Source: CAD feature listing. Evaluate the final solid. Frame: model axes, mm. Face numbers are marked on the shaded views. A direction names the side the tool comes from. Round coordinates to 2 decimals unless told otherwise and drop trailing zeros. Write each loop counter-clockwise with the first axis right and the second up, starting at its lowest first coordinate (ties: lowest second). Pieces come first, ordered by that corner, then holes.
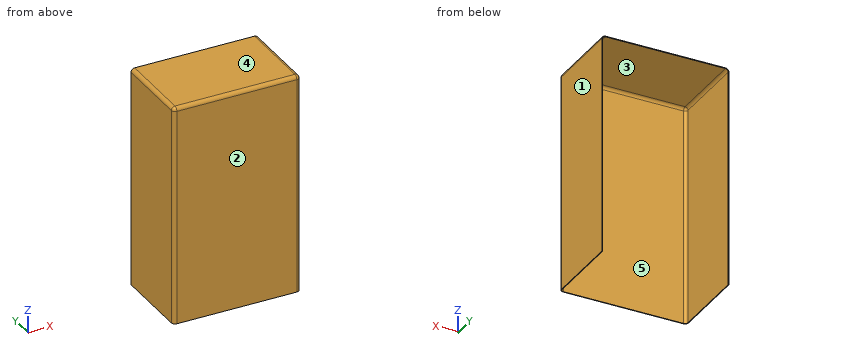
```python
from build123d import *

# Parameters (mm, degrees)
SKETCH_1_W      = 350
SKETCH_1_H      = 220
EXTRUDE_1_DEPTH = 607
FILLET_1_R      = 10
SHELL_1_T       = -2


with BuildPart() as part:
    # 草图1 → 凸台-拉伸1 (new body)
    with BuildSketch(Plane.XY):
        Rectangle(SKETCH_1_W, SKETCH_1_H)
    extrude(amount=EXTRUDE_1_DEPTH)

    # 圆角1
    fillet_1_edges = [part.edges().sort_by_distance(p)[0] for p in [
        (-175, 0, 607),
        (0, -110, 607),
        (175, 0, 607),
        (175, -110, 303.5),
        (-175, -110, 303.5),
    ]]
    fillet(fillet_1_edges, radius=FILLET_1_R)

    # 抽壳1
    shell_1_openings = [part.faces().sort_by_distance(p)[0] for p in [
        (0, 0.060103243, 0),
        (0, 110, 303.439124152),
    ]]
    offset(amount=SHELL_1_T, openings=shell_1_openings, kind=Kind.INTERSECTION)


solid = part.part
```
Q1. Mould query, pull axis X, two halves, no side actions, for the marked faces 1, 2 and 3. Classes: pulls with the +X half, pulls with the -X half, needs draft (parallel to the pull), parting line crosses it, or undercut.
Q2. Section query C-C, the plane x = 58. Output: boundary loops of the cut face in (y, z), and give its area (3 significant figures).
Q3. Set-up query: the marked faces 4 and 5. Return all of +Z, -Z, +X, -X, +Y, -Y with unobstructed straight access to the full face (end or side cutting, diameter ignored); none if empty.
Q4. Pin query (flat end, axial travel): P1, Ø3, axis at x = -42, y = 70, coming from the -Z side; P2, Ø10, axis at x = -66.5, z = 157, coming from the +Y side. Return the tip coordinate at first contact, or that it passes through.
Q5. Section query B-B, the plane z = 331.5. Output: boundary loops of the cut face in (x, y).
Q6. Line query: line 1 (X direction, y = -69.5, z = 495); line 2 (Y direction, x = -77, z = 522.5); line 3 (Z direction, x = -71.5, y = 58). Output: solid intervals per line, ascending.
Q7. Section query A-A, the plane y = -36.5. Output: boundary loops of the cut face in (x, z).
Filled in:
1. face 1: pulls with the +X half
1. face 2: needs draft
1. face 3: undercut
2. outline: (-110, 0) - (-108, 0) - (-108, 597) arc R8 cw to (-100, 605) - (110, 605) - (110, 607) - (-100, 607) arc R10 ccw to (-110, 597) - close
2. area: 1,640 mm2
3. face 4: +Z, +X, -X, +Y, -Y
3. face 5: -Z, +Y
4. P1: stops at z = 605
4. P2: stops at y = -108
5. outline: (-175, -100) arc R10 ccw to (-165, -110) - (165, -110) arc R10 ccw to (175, -100) - (175, 110) - (173, 110) - (173, -100) arc R8 cw to (165, -108) - (-165, -108) arc R8 cw to (-173, -100) - (-173, 110) - (-175, 110) - close
6. line 1: x = -175 to -173, 173 to 175
6. line 2: y = -110 to -108
6. line 3: z = 605 to 607
7. outline: (-175, 0) - (-173, 0) - (-173, 597) arc R8 cw to (-165, 605) - (165, 605) arc R8 cw to (173, 597) - (173, 0) - (175, 0) - (175, 597) arc R10 ccw to (165, 607) - (-165, 607) arc R10 ccw to (-175, 597) - close
